Build history of the part. All positions in model axes, mm. Face numbers are marked on the shaded views. A direction names the side the tool comes from. Coordinates: 2 decimals unless noted, no trailing zeros. Order: outer loops, then holes, each group sorted by start corner. A loop starts at its lowest first (then second) coordinate and runs counter-clockwise, first axis right, second up. Notation, with made-up numbers: M -10,29 L 29,29 A21 cw 29,33 Z; hole C 2,11 d2. An arc over 180 degrees is marked long. Use a Markdown table: item, result. Add a question column.
from build123d import *

# Parameters (mm, degrees)
F0_W         = 127
F0_H         = 76.2
F1_DEPTH     = 6.35
F2_R         = 5.08
F4_W         = 129.3370249418
F4_H         = 77.6022149651
F5_DEPTH     = 6.35
F6_R         = 5.08
F7_DEPTH     = 6.35
F8_R         = 2.38125
F9_DEPTH     = 25.4
F10_DEPTH    = 6.35
F11_T1_DEPTH = 31.75


# Not quite as in the source:
# - a fillet or chamfer that OpenCascade refuses, or shapes differently, is made with other operations: its cross-section is extruded or revolved along the edge and cut away or added


with BuildPart() as f1:
    # F0 (on Top) → F1 (new body)
    with BuildSketch(Plane.XY):
        Rectangle(F0_W, F0_H)
    extrude(amount=F1_DEPTH)

    # F2
    f2_edges = [f1.edges().sort_by_distance(p)[0] for p in [
        (-63.5, 38.1, 3.175),
        (-63.5, -38.1, 3.175),
        (63.5, -38.1, 3.175),
        (63.5, 38.1, 3.175),
    ]]
    fillet(f2_edges, radius=F2_R)

    # F4 (on offset) → F5 (join)
    with BuildSketch(Plane.XY.offset(6.35)):
        Rectangle(F4_W, F4_H)
        Polygon((-57.15, -16.6380591357), (-57.15, 16.6380591357), (-57.15, 31.75), (57.15, 31.75), (57.15, 16.6380591357), (57.15, -16.6380591357), (57.15, -31.75), (-57.15, -31.75), align=None, mode=Mode.SUBTRACT)
    extrude(amount=F5_DEPTH)

    # F6
    f6_edges = [f1.edges().sort_by_distance(p)[0] for p in [
        (-64.668512, -38.801107, 9.525),
        (64.668512, 38.801107, 9.525),
        (64.668512, -38.801107, 9.525),
        (-64.668512, 38.801107, 9.525),
    ]]
    fillet(f6_edges, radius=F6_R)

    # F4 (on offset) → F7 (join)
    with BuildSketch(Plane.XY.offset(6.35)):
        Polygon((-46.2962661107, 12.9479340409), (-46.2962661107, -16.6380591357), (-42.4617134193, -16.6380591357), (-42.4617134193, 12.9479340409), (-32.0123768006, 12.9479340409), (-32.0123768006, 16.3564253222), (-56.7456027293, 16.3564253222), (-56.7456027293, 12.9479340409), align=None)
        Polygon((-27.0440674754, 16.3564253222), (-27.0440674754, -16.6380591357), (-8.6512130402, -16.6380591357), (-8.6512130402, -13.2079037149), (-23.2095147839, -13.2079037149), (-23.2095147839, -1.0687642153), (-9.5322213798, -1.0687642153), (-9.5322213798, 2.3180629265), (-23.2095147839, 2.3180629265), (-23.2095147839, 12.9479340409), (-8.6512130402, 12.9479340409), (-8.6512130402, 16.3564253222), align=None)
        with BuildLine():
            Line((15.9701099418, 16.6380591357), (10.0159430302, 16.6380591357))
            add(Edge.make_bspline(
                [(4.3581027293, 14.7496683093), (6.8753977724, 16.2014683592), (10.0159430302, 16.6380591357)],
                knots=[0, 0, 0, 0.6992762354, 0.6992762354, 0.6992762354], degree=2))
            add(Edge.make_bspline(
                [(-1.1481993935, 8.8389689158), (0.7582448825, 12.6735216073), (4.3581027293, 14.7496683093)],
                knots=[0, 0, 0, 1, 1, 1], degree=2))
            add(Edge.make_bspline(
                [(-3.0546436694, -0.0938779378), (-3.0546436694, 5.0044162244), (-1.1481993935, 8.8389689158)],
                knots=[0, 0, 0, 1, 1, 1], degree=2))
            add(Edge.make_bspline(
                [(0.9062831691, -12.6663002274), (-3.0546436694, -8.2395943897), (-3.0546436694, -0.0938779378)],
                knots=[0, 0, 0, 1, 1, 1], degree=2))
            add(Edge.make_bspline(
                [(7.8235797826, -16.6380591357), (3.5974055182, -15.6738809021), (0.9062831691, -12.6663002274)],
                knots=[0.3205826669, 0.3205826669, 0.3205826669, 1, 1, 1], degree=2))
            Line((7.8235797826, -16.6380591357), (17.5614415983, -16.6380591357))
            add(Edge.make_bspline(
                [(20.6170394238, -15.8003790751), (19.2218518782, -16.326144487), (17.5614415983, -16.6380591357)],
                knots=[0, 0, 0, 0.406741787, 0.406741787, 0.406741787], degree=2))
            Line((20.6170394238, -15.8003790751), (20.6170394238, -12.4424374526))
            add(Edge.make_bspline(
                [(12.7385140258, -13.6845147839), (16.1903335861, -13.6845147839), (20.6170394238, -12.4424374526)],
                knots=[0, 0, 0, 1, 1, 1], degree=2))
            add(Edge.make_bspline(
                [(4.0836902957, -10.1496493556), (7.1202805155, -13.6845147839), (12.7385140258, -13.6845147839)],
                knots=[0, 0, 0, 1, 1, 1], degree=2))
            add(Edge.make_bspline(
                [(1.0471000758, -0.1444275967), (1.0471000758, -6.6147839272), (4.0836902957, -10.1496493556)],
                knots=[0, 0, 0, 1, 1, 1], degree=2))
            add(Edge.make_bspline(
                [(4.1956216831, 9.7741376042), (1.0471000758, 6.1526156179), (1.0471000758, -0.1444275967)],
                knots=[0, 0, 0, 1, 1, 1], degree=2))
            add(Edge.make_bspline(
                [(12.7818423048, 13.3956595906), (7.3441432904, 13.3956595906), (4.1956216831, 9.7741376042)],
                knots=[0, 0, 0, 1, 1, 1], degree=2))
            add(Edge.make_bspline(
                [(20.2776345716, 11.6408642911), (16.5297384382, 13.3956595906), (12.7818423048, 13.3956595906)],
                knots=[0, 0, 0, 1, 1, 1], degree=2))
            Line((20.2776345716, 11.6408642911), (21.9024450341, 14.9338134951))
            add(Edge.make_bspline(
                [(15.9701099418, 16.6380591357), (19.2412217115, 16.2297995741), (21.9024450341, 14.9338134951)],
                knots=[0.3150184776, 0.3150184776, 0.3150184776, 1, 1, 1], degree=2))
        make_face()
        with BuildLine():
            Line((27.8167551175, -16.6380591357), (36.9590219864, -16.6380591357))
            add(Edge.make_bspline(
                [(49.7192001516, -12.3160633055), (45.285272934, -16.6380591357), (36.9590219864, -16.6380591357)],
                knots=[0, 0, 0, 1, 1, 1], degree=2))
            add(Edge.make_bspline(
                [(54.1531273692, 0.173313116), (54.1531273692, -7.9940674754), (49.7192001516, -12.3160633055)],
                knots=[0, 0, 0, 1, 1, 1], degree=2))
            add(Edge.make_bspline(
                [(49.8889025777, 12.0922005307), (54.1531273692, 7.8279757392), (54.1531273692, 0.173313116)],
                knots=[0, 0, 0, 1, 1, 1], degree=2))
            add(Edge.make_bspline(
                [(37.926686884, 16.3564253222), (45.6246777862, 16.3564253222), (49.8889025777, 12.0922005307)],
                knots=[0, 0, 0, 1, 1, 1], degree=2))
            Line((37.926686884, 16.3564253222), (27.8167551175, 16.3564253222))
            Line((27.8167551175, 16.3564253222), (27.8167551175, -16.6380591357))
        make_face()
        with BuildLine():
            add(Edge.make_bspline(
                [(50.094711903, 0.0361068992), (50.094711903, 6.4920204701), (46.8559230478, 9.7633055345)],
                knots=[0, 0, 0, 1, 1, 1], degree=2))
            add(Edge.make_bspline(
                [(46.6392816528, -9.9474507202), (50.094711903, -6.5714556482), (50.094711903, 0.0361068992)],
                knots=[0, 0, 0, 1, 1, 1], degree=2))
            add(Edge.make_bspline(
                [(36.323540561, -13.3234457923), (43.1838514026, -13.3234457923), (46.6392816528, -9.9474507202)],
                knots=[0, 0, 0, 1, 1, 1], degree=2))
            Line((36.323540561, -13.3234457923), (31.6513078089, -13.3234457923))
            Line((31.6513078089, -13.3234457923), (31.6513078089, 13.0345905989))
            Line((31.6513078089, 13.0345905989), (37.2262130402, 13.0345905989))
            add(Edge.make_bspline(
                [(46.8559230478, 9.7633055345), (43.6171341926, 13.0345905989), (37.2262130402, 13.0345905989)],
                knots=[0, 0, 0, 1, 1, 1], degree=2))
        make_face(mode=Mode.SUBTRACT)
    extrude(amount=F7_DEPTH)

    # F8 (on face) → F9 (cut)
    with BuildSketch(Plane(origin=(0, 0, 0), x_dir=(1, 0, 0), z_dir=(0, 0, -1))):
        with Locations((-50.8, 25.4)):
            Circle(F8_R)
        with Locations((-50.8, -25.4)):
            Circle(F8_R)
        with Locations((50.8, -25.4)):
            Circle(F8_R)
        with Locations((50.8, 25.4)):
            Circle(F8_R)
    extrude(amount=-F9_DEPTH, mode=Mode.SUBTRACT)

    # F4 (on offset) → F10 (join)
    with BuildSketch(Plane.XY.offset(6.35)):
        Rectangle(F4_W, F4_H)
        Polygon((-57.15, -16.6380591357), (-57.15, 16.6380591357), (-57.15, 31.75), (57.15, 31.75), (57.15, 16.6380591357), (57.15, -16.6380591357), (57.15, -31.75), (-57.15, -31.75), align=None, mode=Mode.SUBTRACT)
    extrude(amount=-F10_DEPTH)

    # F11: fillet of radius 5.08 on 4 edges, made by hand

    # F11_s2 → F11_t1 (cut)
    with BuildSketch(Plane.XY.offset(-12.7)):
        with BuildLine():
            ThreePointArc((-64.6685124709, 33.7211074825), (-63.1806149193, 37.313209931), (-59.5885124709, 38.8011074825))
            Line((-59.5885124709, 38.8011074825), (-64.6685124709, 38.8011074825))
            Line((-64.6685124709, 38.8011074825), (-64.6685124709, 33.7211074825))
        make_face()
        with BuildLine():
            ThreePointArc((-59.5885124709, -38.8011074825), (-63.1806149193, -37.313209931), (-64.6685124709, -33.7211074825))
            Line((-64.6685124709, -33.7211074825), (-64.6685124709, -38.8011074825))
            Line((-64.6685124709, -38.8011074825), (-59.5885124709, -38.8011074825))
        make_face()
        with BuildLine():
            ThreePointArc((59.5885124709, -38.8011074825), (63.1806149193, -37.313209931), (64.6685124709, -33.7211074825))
            Line((64.6685124709, -33.7211074825), (64.6685124709, -38.8011074825))
            Line((64.6685124709, -38.8011074825), (59.5885124709, -38.8011074825))
        make_face()
        with BuildLine():
            ThreePointArc((64.6685124709, 33.7211074825), (63.1806149193, 37.313209931), (59.5885124709, 38.8011074825))
            Line((59.5885124709, 38.8011074825), (64.6685124709, 38.8011074825))
            Line((64.6685124709, 38.8011074825), (64.6685124709, 33.7211074825))
        make_face()
    extrude(amount=F11_T1_DEPTH, mode=Mode.SUBTRACT)


solid = f1.part
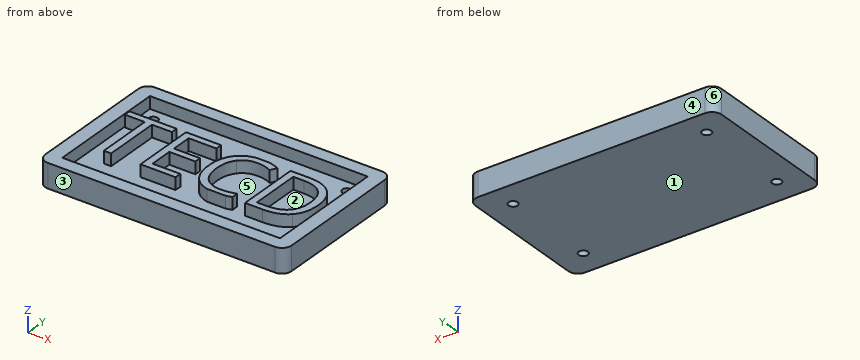
(1) Mould opens along Y. For the marked faces 1, 2, 3 and 4 say: released by +Y, released by -Y, zero draft, split by the parting line, or undercut.
(2) Which spindle directions (+Z, -Z, +X, -X, +Y, -Y) get a long thin tool onto all of the face, cutting with end or side? Do the marked faces 5 and 6. Say none if no direction does.
(3) Slice it at A-A on y = 25.4. Give the cut face in (x, z).
(4) Drop flat-ended pins along their axis: P1, Ø6, axis at x = -37.5, y = 8.5, coming from the +Z side; P2, Ø4, axis at x = -50.8, y = -25.4, coming from the +Z side. Give the stop position or say it passes through.
(5) Drill centre lines: line 1 along X through (y, z) = (-25.4, 4); line 2 along Y through (x, z) = (-25, 7.25); line 3 along X through (y, z) = (23.5, 10.5). Where is each one in solid material? Low to high. Write a range as from..to.
(6) Slice it at B-B on x = -50.8. Give the cut face in (y, z).
(7) Slice it at C-C on z = 8. State how many separate pieces and enclosed holes the cut face has, and give its area (3 significant figures).
Solutions:
| question | item | result |
|---|---|---|
| 1 | face 1 | zero draft |
| 1 | face 2 | undercut |
| 1 | face 3 | released by -Y |
| 1 | face 4 | released by +Y |
| 2 | face 5 | +Z |
| 2 | face 6 | +Z, -Z, -X, +Y |
| 3 | outline | M -64.67,0 L -53.18,0 L -53.18,6.35 L -57.15,6.35 L -57.15,12.7 L -64.67,12.7 Z; M -48.42,0 L 48.42,0 L 48.42,6.35 L -48.42,6.35 Z; M 53.18,0 L 64.67,0 L 64.67,12.7 L 57.15,12.7 L 57.15,6.35 L 53.18,6.35 Z |
| 4 | P1 | z = 6.35 |
| 4 | P2 | through |
| 5 | line 1 | -64.67..-53.18, -48.42..48.42, 53.18..64.67 |
| 5 | line 2 | -38.8..-31.75, -16.64..16.36, 31.75..38.8 |
| 5 | line 3 | -64.67..-57.15, 57.15..64.67 |
| 6 | outline | M -38.8,0 L -27.78,0 L -27.78,6.35 L -31.75,6.35 L -31.75,12.7 L -38.8,12.7 Z; M -23.02,0 L 23.02,0 L 23.02,6.35 L 16.36,6.35 L 16.36,12.7 L 12.95,12.7 L 12.95,6.35 L -23.02,6.35 Z; M 27.78,0 L 38.8,0 L 38.8,12.7 L 31.75,12.7 L 31.75,6.35 L 27.78,6.35 Z |
| 7 | separate pieces | 5 |
| 7 | enclosed holes | 2 |
| 7 | area | 3,810 mm² |
